The listing builds one solid part. Answer for the finished solid, in the listing's coordinates (mm). A direction names the side the tool comes from. Coordinates: 2 decimals unless noted, no trailing zeros. Order: outer loops, then holes, each group sorted by start corner. A loop starts at its lowest first (then second) coordinate and runs counter-clockwise, first axis right, second up. Notation, with made-up numbers: (57.25, -14.75) - (78.25, -14.75) arc R25 ccw to (78.25, 24.25) - close; hole circle Ø6 at (27.5, -22). An arc over 180 degrees is marked (long way). Use one line per item in the form item = value. Start each with the question number.
Item 1: A tool of negligible diameter and unlimited length cuts with its end or side. For faces 5 (the flat face through (23.66, 138.15, -88.2)), 6 (the flat face through (-23.01, 138.15, -88.47)), 7 (the flat face through (0, 73, 84.5)), from which of +Z, -Z, +X, -X, +Y, -Y can it reach the whole face along a straight path? Write none if from no direction.
Item 2: Section D-D, the plane y = 151 is taken. Write down the section's boundary in (x, z), and give its area (3 significant figures).
Item 3: Section A-A, the plane z = 96.5 is taken. Write down the section's boundary in (x, y), and give its area (4 significant figures).
Item 4: Consider line 1 along X through (y, z) = (128, -78.5); line 2 along Z through (x, y) = (-46, 38); line 3 along Y through (x, z) = (51.5, 98). Determine where each line is inside the solid, lowest interval first. Write a range as [from, to].
Item 5: Section C-C, the plane x = 16.5 is taken. Write down the section's boundary in (y, z).
Item 6: Each of these flat-tipped pins is pushed along its axis until it touches: pin 1 Ø3 at (x, z) = (118, 95.5) entering from +Y; pin 2 Ø22.5 at (x, z) = (-14, 70) entering from +Y; pin 3 Ø12 at (y, z) = (48.5, -111.5) entering from +X. Where does it stop, or does it pass through?
Item 7: The mould has two halves that part along Z. Classify faces 1 (the flat face through (-62.5, 27, 104)), 2 (the flat face through (47, 27, 59)), 3 (the flat face through (-87.27, 38.45, 3.56)), 4 (the flat face through (0, 85, 39.5)): released by +Z, released by -Z, zero draft, split by the parting line, or undercut.
Item 8: Section B-B, the plane y = 32 is taken. Write down the section's boundary in (x, z).
from build123d import *

# Parameters (mm, degrees)
SKETCH_1_W      = 300
SKETCH_1_H      = 300
EXTRUDE_1_DEPTH = 15
EXTRUDE_2_DEPTH = 78
EXTRUDE_3_DEPTH = 200
SKETCH_4_W      = 125
SKETCH_4_H      = 88
EXTRUDE_4_DEPTH = 54
SKETCH_5_W      = 65
SKETCH_5_H      = 45
EXTRUDE_5_DEPTH = 92


with BuildPart() as part:
    # 草图1 → 凸台-拉伸1 (new body)
    with BuildSketch(Plane(origin=(0, 0, 0), x_dir=(1, 0, 0), z_dir=(0, 1, 0))):
        Rectangle(SKETCH_1_W, SKETCH_1_H)
    extrude(amount=-EXTRUDE_1_DEPTH)

    # 草图2 → 凸台-拉伸2 (add)
    with BuildSketch(Plane(origin=(0, 0, 0), x_dir=(1, 0, 0), z_dir=(0, 1, 0))):
        Polygon((102, 32), (72.124891681, 104.124891681), (0, 134), (-72.124891681, 104.124891681), (-102, 32), (-72.124891681, -40.124891681), (0, -70), (72.124891681, -40.124891681), align=None)
    extrude(amount=EXTRUDE_2_DEPTH)

    # 草图3 → 凸台-拉伸3 (add)
    with BuildSketch(Plane(origin=(0, 0, 0), x_dir=(1, 0, 0), z_dir=(0, 1, 0))):
        Polygon((66, 32), (46.669047558, 78.669047558), (0, 98), (-46.669047558, 78.669047558), (-66, 32), (-46.669047558, -14.669047558), (0, -34), (46.669047558, -14.669047558), align=None)
    extrude(amount=EXTRUDE_3_DEPTH)

    # 草图4 → 凸台-拉伸4 (add)
    with BuildSketch(Plane(origin=(0, 0, 0), x_dir=(1, 0, 0), z_dir=(0, 1, 0))):
        with Locations((0, -103)):
            Rectangle(SKETCH_4_W, SKETCH_4_H)
    extrude(amount=EXTRUDE_4_DEPTH)

    # 草图5 → 凸台-拉伸5 (add)
    with BuildSketch(Plane(origin=(0, 0, 0), x_dir=(1, 0, 0), z_dir=(0, 1, 0))):
        with Locations((0, -62)):
            Rectangle(SKETCH_5_W, SKETCH_5_H)
    extrude(amount=EXTRUDE_5_DEPTH)


solid = part.part
Response:
q1.face_5 = -Z, +X, +Y
q1.face_6 = -Z, -X, +Y
q1.face_7 = +Z, +X, -X, +Y
q2.outline = (-66, -32) - (-46.67, -78.67) - (0, -98) - (46.67, -78.67) - (66, -32) - (46.67, 14.67) - (0, 34) - (-46.67, 14.67) - close
q2.area = 12,300 mm2
q3.outline = (-150, -15) - (150, -15) - (150, 0) - (62.5, 0) - (62.5, 54) - (-62.5, 54) - (-62.5, 0) - (-150, 0) - close
q3.area = 11,250 mm2
q4.line_1 = [-46.74, 46.74]
q4.line_2 = [-114.95, 50.95], [59, 147]
q4.line_3 = [-15, 54]
q5.outline = (-15, -150) - (0, -150) - (0, -127.17) - (78, -127.17) - (78, -91.17) - (200, -91.17) - (200, 27.17) - (78, 27.17) - (78, 39.5) - (92, 39.5) - (92, 84.5) - (54, 84.5) - (54, 147) - (0, 147) - (0, 150) - (-15, 150) - close
q6.pin_1 = 0
q6.pin_2 = 92
q6.pin_3 = 68.81
q7.face_1 = zero draft
q7.face_2 = undercut
q7.face_3 = released by +Z
q7.face_4 = undercut
q8.outline = (-102, -32) - (-72.12, -104.12) - (0, -134) - (72.12, -104.12) - (102, -32) - (72.12, 40.12) - (32.5, 56.54) - (32.5, 59) - (62.5, 59) - (62.5, 147) - (-62.5, 147) - (-62.5, 59) - (-32.5, 59) - (-32.5, 56.54) - (-72.12, 40.12) - close
